Could you check a few things on this model? Use its own coordinates, in mm. Face numbers are marked on the shaded views. A direction names the side the tool comes from. Give positions to 0.01 mm unless a question says otherwise; leave off trailing zeros. Order: outer loops, then holes, each group sorted by start corner. A loop starts at its lowest first (then second) coordinate and runs counter-clockwise, first axis right, second up. Notation, with made-up numbers: (18, 39.25) -> (34, 39.25) arc R7 cw to (34, 43.25) -> close; hole circle Ø8 at (66.25, 15.5). An arc over 180 degrees is marked (long way). Answer as CSV lines item,"result". Start each with the question number.
(1) On a 3-axis mill with a long thin cutter (end or side, diameter ignored), from which of +Z, -Z, +X, -X, +Y, -Y can I reach the whole of each face in a straight line? I mean the marked faces 5, 6, 7 and 8. Say none if no direction works.
(2) I want a section at B-B (z = -29). Please give me the cut outline in (x, y).
(3) I want a section at A-A (x = 31.75). Please give me the cut outline in (y, z).
(4) We'd pull the mould along X, two halves only. Please class the marked faces 1, 2, 3 and 4: released by +X, released by -X, zero draft, split by the parting line, or undercut.
(5) I want a section at C-C (y = -11.5). Please give me the cut outline in (x, z), plus the area to 3 significant figures.
(6) Will these pins go through, and if not, where does the flat tip stop? pin 1 Ø6 at (x, y) = (31.5, -9.5) entering from +Z; pin 2 Ø6 at (x, y) = (29, -7) entering from +Z; pin 3 Ø5 at (x, z) = (20, -11.5) entering from -Y.
(7) I need wall thicknesses on L1, parallel to Z at x = 34, y = -6.3; L2, parallel to Z at x = 33, y = -7.25; L3, parallel to Y at x = 28, z = -13.75. Which ranges of each line are inside material? Lowest first, please.
(8) I want a section at D-D (x = 18). Please give me the cut outline in (y, z), plus the area to 3 significant figures.
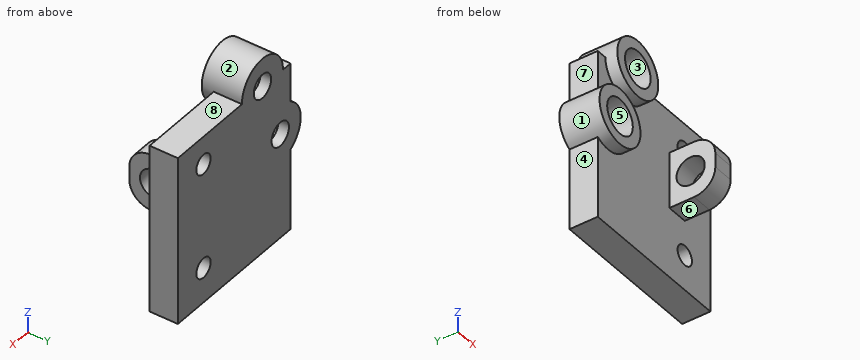
```python
from build123d import *

# Parameters (mm, degrees)
CYLINDER267_R               = 2
CYLINDER267_DEPTH           = 10
CYLINDER267_PITCH_ANGLE     = 90
BOX001027045199_W           = 3
BOX001027045199_H           = 8
BOX001027045199_DEPTH       = 8
FILLET045_R                 = 3
CUT240_ROLL_ANGLE           = 90
CYLINDER257_R               = 2.5
CYLINDER257_DEPTH           = 30
CYLINDER257_ROLL_ANGLE      = 90
CYLINDER258_R               = 1.7
CYLINDER258_DEPTH           = 50
CYLINDER258_ROLL_ANGLE      = 90
CYLINDER262_R               = 1.7
CYLINDER262_DEPTH           = 30
CYLINDER262_ROLL_ANGLE      = 89.999963
CYLINDER262_PITCH_ANGLE     = 11.999988
CYLINDER262_PLACEMENT_ANGLE = -4e-06
CYLINDER259_R               = 2.5
CYLINDER259_DEPTH           = 20
CYLINDER259_ROLL_ANGLE      = 89.999963
CYLINDER259_PITCH_ANGLE     = 11.999988
CYLINDER259_PLACEMENT_ANGLE = -4e-06
CYLINDER231_R               = 1.4
CYLINDER231_DEPTH           = 20
CYLINDER231_ROLL_ANGLE      = 90
CYLINDER230_R               = 1.4
CYLINDER230_DEPTH           = 20
CYLINDER230_ROLL_ANGLE      = 90
BOX001027045174_W           = 22
BOX001027045174_H           = 4
BOX001027045174_DEPTH       = 24
CYLINDER260_R               = 4
CYLINDER260_DEPTH           = 5.7
CYLINDER260_ROLL_ANGLE      = 90
CYLINDER261_R               = 4
CYLINDER261_DEPTH           = 5.7
CYLINDER261_ROLL_ANGLE      = 90
CYLINDER261_PITCH_ANGLE     = 12


with BuildPart() as cylinder285:
    # Cylinder267 → Cylinder267 (new body)
    with BuildSketch(Plane.XY):
        Circle(CYLINDER267_R)
    extrude(amount=CYLINDER267_DEPTH)


with BuildPart() as cylinder285_1:
    # Cylinder267 pitch: moved
    add(cylinder285.part.rotate(Axis((0, 0, 0), (0, 1, 0)), CYLINDER267_PITCH_ANGLE))


with BuildPart() as cylinder285_2:
    # Cylinder267 placement: moved
    add(cylinder285_1.part.moved(Location((-3, 4, 4.5))))


with BuildPart() as cut240:
    # Box001027045199 → Box001027045199 (new body)
    with BuildSketch(Plane.XY):
        with Locations((1.5, 4)):
            Rectangle(BOX001027045199_W, BOX001027045199_H)
    extrude(amount=BOX001027045199_DEPTH)

    # Fillet045
    fillet045_edges = [cut240.edges().sort_by_distance(p)[0] for p in [
        (1.5, 0, 8),
        (1.5, 8, 8),
    ]]
    fillet(fillet045_edges, radius=FILLET045_R)

    # Cut240: cut Cylinder285
    add(cylinder285_2.part, mode=Mode.SUBTRACT)


with BuildPart() as cut240_1:
    # Cut240 roll: moved
    add(cut240.part.rotate(Axis((0, 0, 0), (1, 0, 0)), CUT240_ROLL_ANGLE))


with BuildPart() as cut240_2:
    # Cut240 placement: moved
    add(cut240_1.part.moved(Location((31, -7, -24))))


with BuildPart() as cylinder275:
    # Cylinder257 → Cylinder257 (new body)
    with BuildSketch(Plane.XY):
        Circle(CYLINDER257_R)
    extrude(amount=CYLINDER257_DEPTH)


with BuildPart() as cylinder275_1:
    # Cylinder257 roll: moved
    add(cylinder275.part.rotate(Axis((0, 0, 0), (1, 0, 0)), CYLINDER257_ROLL_ANGLE))


with BuildPart() as cylinder275_2:
    # Cylinder257 placement: moved
    add(cylinder275_1.part.moved(Location((23, 36, -19))))


with BuildPart() as fusion112142:
    # Cylinder258 → Cylinder258 (new body)
    with BuildSketch(Plane.XY):
        Circle(CYLINDER258_R)
    extrude(amount=CYLINDER258_DEPTH)


with BuildPart() as fusion112142_1:
    # Cylinder258 roll: moved
    add(fusion112142.part.rotate(Axis((0, 0, 0), (1, 0, 0)), CYLINDER258_ROLL_ANGLE))


with BuildPart() as fusion112142_2:
    # Cylinder258 placement: moved
    add(fusion112142_1.part.moved(Location((23, 18, -19))))

    # Fusion112142: union Cylinder275
    add(cylinder275_2.part)


with BuildPart() as part_mirroring016:
    # Part__Mirroring016: instance of Fusion112142
    add(fusion112142_2.part.mirror(Plane(origin=(0, 0, 0), x_dir=(1, 0, 0), z_dir=(0, 1, 0))))


with BuildPart() as part_mirroring016_1:
    # Part__Mirroring016 placement: moved
    add(part_mirroring016.part.moved(Location((-4, 0, 0))))


with BuildPart() as cylinder280:
    # Cylinder262 → Cylinder262 (new body)
    with BuildSketch(Plane.XY):
        Circle(CYLINDER262_R)
    extrude(amount=CYLINDER262_DEPTH)


with BuildPart() as cylinder280_1:
    # Cylinder262 roll: moved
    add(cylinder280.part.rotate(Axis((0, 0, 0), (1, 0, 0)), CYLINDER262_ROLL_ANGLE))


with BuildPart() as cylinder280_2:
    # Cylinder262 pitch: moved
    add(cylinder280_1.part.rotate(Axis((0, 0, 0), (0, 1, 0)), CYLINDER262_PITCH_ANGLE))


with BuildPart() as cylinder280_3:
    # Cylinder262 placement: moved
    add(cylinder280_2.part.moved(Location((22.4783, 12.2, -9.9062))).rotate(Axis((22.4783, 12.2, -9.9062), (0, 0, 1)), CYLINDER262_PLACEMENT_ANGLE))


with BuildPart() as fusion112149:
    # Cylinder259 → Cylinder259 (new body)
    with BuildSketch(Plane.XY):
        Circle(CYLINDER259_R)
    extrude(amount=CYLINDER259_DEPTH)


with BuildPart() as fusion112149_1:
    # Cylinder259 roll: moved
    add(fusion112149.part.rotate(Axis((0, 0, 0), (1, 0, 0)), CYLINDER259_ROLL_ANGLE))


with BuildPart() as fusion112149_2:
    # Cylinder259 pitch: moved
    add(fusion112149_1.part.rotate(Axis((0, 0, 0), (0, 1, 0)), CYLINDER259_PITCH_ANGLE))


with BuildPart() as fusion112149_3:
    # Cylinder259 placement: moved
    add(fusion112149_2.part.moved(Location((22.4783, -6, -9.9062))).rotate(Axis((22.4783, -6, -9.9062), (0, 0, 1)), CYLINDER259_PLACEMENT_ANGLE))

    # Fusion112146: union Cylinder280
    add(cylinder280_3.part)

    # Fusion112149: union Part__Mirroring016
    add(part_mirroring016_1.part)


with BuildPart() as m3_tap006:
    # Cylinder231 → Cylinder231 (new body)
    with BuildSketch(Plane.XY):
        Circle(CYLINDER231_R)
    extrude(amount=CYLINDER231_DEPTH)


with BuildPart() as m3_tap006_1:
    # Cylinder231 roll: moved
    add(m3_tap006.part.rotate(Axis((0, 0, 0), (1, 0, 0)), CYLINDER231_ROLL_ANGLE))


with BuildPart() as m3_tap006_2:
    # Cylinder231 placement: moved
    add(m3_tap006_1.part.moved(Location((34, 5, -29))))


with BuildPart() as fusion112123:
    # Cylinder230 → Cylinder230 (new body)
    with BuildSketch(Plane.XY):
        Circle(CYLINDER230_R)
    extrude(amount=CYLINDER230_DEPTH)


with BuildPart() as fusion112123_1:
    # Cylinder230 roll: moved
    add(fusion112123.part.rotate(Axis((0, 0, 0), (1, 0, 0)), CYLINDER230_ROLL_ANGLE))


with BuildPart() as fusion112123_2:
    # Cylinder230 placement: moved
    add(fusion112123_1.part.moved(Location((34, 5, -14))))

    # Fusion112123: union M3-tap006
    add(m3_tap006_2.part)


with BuildPart() as cut234:
    # Box001027045174 → Box001027045174 (new body)
    with BuildSketch(Plane(origin=(17, -8.5, -34), x_dir=(1, 0, 0), z_dir=(0, 0, 1))):
        with Locations((11, 2)):
            Rectangle(BOX001027045174_W, BOX001027045174_H)
    extrude(amount=BOX001027045174_DEPTH)

    # Cut234: cut Fusion112123
    add(fusion112123_2.part, mode=Mode.SUBTRACT)


with BuildPart() as cylinder278:
    # Cylinder260 → Cylinder260 (new body)
    with BuildSketch(Plane.XY):
        Circle(CYLINDER260_R)
    extrude(amount=CYLINDER260_DEPTH)


with BuildPart() as cylinder278_1:
    # Cylinder260 roll: moved
    add(cylinder278.part.rotate(Axis((0, 0, 0), (1, 0, 0)), CYLINDER260_ROLL_ANGLE))


with BuildPart() as cylinder278_2:
    # Cylinder260 placement: moved
    add(cylinder278_1.part.moved(Location((19, 10.2, -19))))


with BuildPart() as part_mirroring017:
    # Part__Mirroring017: instance of Cylinder278
    add(cylinder278_2.part.mirror(Plane(origin=(0, 0, 0), x_dir=(1, 0, 0), z_dir=(0, 1, 0))))


with BuildPart() as cylinder279:
    # Cylinder261 → Cylinder261 (new body)
    with BuildSketch(Plane.XY):
        Circle(CYLINDER261_R)
    extrude(amount=CYLINDER261_DEPTH)


with BuildPart() as cylinder279_1:
    # Cylinder261 roll: moved
    add(cylinder279.part.rotate(Axis((0, 0, 0), (1, 0, 0)), CYLINDER261_ROLL_ANGLE))


with BuildPart() as cylinder279_2:
    # Cylinder261 pitch: moved
    add(cylinder279_1.part.rotate(Axis((0, 0, 0), (0, 1, 0)), CYLINDER261_PITCH_ANGLE))


with BuildPart() as cylinder279_3:
    # Cylinder261 placement: moved
    add(cylinder279_2.part.moved(Location((22.478298, 10.2, -9.906203))))


with BuildPart() as clamp_plate:
    # Part__Mirroring018: instance of Cylinder279
    add(cylinder279_3.part.mirror(Plane(origin=(0, 0, 0), x_dir=(1, 0, 0), z_dir=(0, 1, 0))))

    # Fusion112144: union Part__Mirroring017
    add(part_mirroring017.part)

    # Fusion112145: union Cut234
    add(cut234.part)

    # Cut236: cut Fusion112149
    add(fusion112149_3.part, mode=Mode.SUBTRACT)

    # Fusion112155: union Cut240
    add(cut240_2.part)


solid = clamp_plate.part
```
Final values:
1,face 5,"-Y"
1,face 6,"-Z, +X, -X, -Y"
1,face 7,"+Z, -X, +Y, -Y"
1,face 8,"+Z, +X, +Y, -Y"
2,outline,"(17, -8.5) -> (32.6, -8.5) -> (32.6, -4.5) -> (17, -4.5) -> close; (35.4, -8.5) -> (39, -8.5) -> (39, -4.5) -> (35.4, -4.5) -> close"
3,outline,"(-15, -21) arc R3 ccw to (-12, -24) -> (-8.5, -24) -> (-8.5, -34) -> (-4.5, -34) -> (-4.5, -10) -> (-8.5, -10) -> (-8.5, -16) -> (-12, -16) arc R3 ccw to (-15, -19) -> close; hole circle Ø4 at (-11.5, -20)"
4,face 1,"undercut"
4,face 2,"split by the parting line"
4,face 3,"undercut"
4,face 4,"released by -X"
5,outline,"(31, -24) -> (34, -24) -> (34, -22) -> (31, -22) -> close; (31, -18) -> (34, -18) -> (34, -16) -> (31, -16) -> close"
5,area,"12.0 mm²"
6,pin 1,"z = -10"
6,pin 2,"z = -8.01"
6,pin 3,"y = -10.2"
7,L1,"-34 to -30.4, -27.6 to -15.4, -12.6 to -10"
7,L2,"-34 to -29.98, -28.02 to -14.98, -13.02 to -10"
7,L3,"-8.5 to -4.5"
8,outline,"(-10.2, -22.87) -> (-8.5, -22.87) -> (-8.5, -34) -> (-4.5, -34) -> (-4.5, -20.37) -> (-6, -20.37) -> (-6, -21.29) -> (-10.2, -21.29) -> close; (-10.2, -16.71) -> (-6, -16.71) -> (-6, -17.63) -> (-4.5, -17.63) -> (-4.5, -10) -> (-8.5, -10) -> (-8.5, -15.13) -> (-10.2, -15.13) -> close"
8,area,"85.8 mm²"
